Can you work these out from the model? Positions are in its coordinate system, mm. A direction names the side the tool comes from. Give positions to 0.01 mm unless a question says otherwise; leave off trailing zeros. Order: outer loops, then holes, each group sorted by start corner. A loop starts at its lowest first (then second) coordinate and runs counter-clockwise, first axis right, second up. Notation, with made-up numbers: (78.5, 6) -> (91.5, 6) arc R30 ccw to (91.5, 29) -> close; hole circle Ø4 at (-18.5, 7.5). An arc over 180 degrees is marked (long way). Answer as CSV lines item,"result".
```python
from build123d import *

# Parameters (mm, degrees)
SKETCH1_W           = 300.101088838
SKETCH1_H           = 6.35
BOSS_EXTRUDE1_DEPTH = 38.1
SKETCH2_W           = 40
SKETCH2_H           = 20
CUT_EXTRUDE1_DEPTH  = 7.35


with BuildPart() as part:
    # Sketch1 → Boss-Extrude1 (new body)
    with BuildSketch(Plane.XY.offset(-6.35)):
        with Locations((245.392650566, 49.505069687)):
            Rectangle(SKETCH1_W, SKETCH1_H)
    extrude(amount=BOSS_EXTRUDE1_DEPTH)

    # Sketch2 → Cut-Extrude1 (cut, through all)
    with BuildSketch(Plane(origin=(0, 52.680069687, 0), x_dir=(1, 0, 0), z_dir=(0, 1, 0))):
        with Locations((325.026890103, -12.7)):
            Rectangle(SKETCH2_W, SKETCH2_H)
    extrude(amount=-CUT_EXTRUDE1_DEPTH, mode=Mode.SUBTRACT)


solid = part.part
```
Item 1: Imagine slicing it at B-B, the plane x = 327. Please give me the cut outline in (y, z), then the cut area to 3 significant figures.
Numbers:
outline,"(46.33, -6.35) -> (52.68, -6.35) -> (52.68, 2.7) -> (46.33, 2.7) -> close; (46.33, 22.7) -> (52.68, 22.7) -> (52.68, 31.75) -> (46.33, 31.75) -> close"
area,"115 mm²"
Item 2: For faces 5 (the flat face through (345.027, 50, 13)), 6 (the flat face through (243, 52.68, 12)), which set-ups out of +Z, -Z, +X, -X, +Y, -Y let a thin tool reach every point of the face, with its end or its side?
Numbers:
face 5,"+Y, -Y"
face 6,"+Z, -Z, +X, -X, +Y"
Item 3: Please list where these lines run through material, in increasing order: line 1 along X through (y, z) = (51.5, 10); line 2 along Z through (x, y) = (315, 47).
Numbers:
line 1,"x = 95.34 to 305.03, 345.03 to 395.44"
line 2,"z = -6.35 to 2.7, 22.7 to 31.75"
Item 4: We'd pull the mould along Z, two halves only. Please class faces 1 (the flat face through (243, 50, 31.75)), 2 (the flat face through (243, 50, -6.35)), 3 (the flat face through (305.027, 50, 13)), 4 (the flat face through (243, 46.33, 12)): released by +Z, released by -Z, zero draft, split by the parting line, or undercut.
Numbers:
face 1,"released by +Z"
face 2,"released by -Z"
face 3,"undercut"
face 4,"zero draft"
Item 5: Imagine slicing it at A-A, the plane z = 7.5. Please give me the cut outline in (x, y), then the cut area to 3 significant figures.
Numbers:
outline,"(95.34, 46.33) -> (305.03, 46.33) -> (305.03, 52.68) -> (95.34, 52.68) -> close; (345.03, 46.33) -> (395.44, 46.33) -> (395.44, 52.68) -> (345.03, 52.68) -> close"
area,"1,650 mm²"
Item 6: Imagine slicing it at C-C, the plane y = 47.5. Please give me the cut outline in (x, z), then the cut area to 3 significant figures.
Numbers:
outline,"(95.34, -6.35) -> (395.44, -6.35) -> (395.44, 31.75) -> (95.34, 31.75) -> close; hole (305.03, 2.7) -> (345.03, 2.7) -> (345.03, 22.7) -> (305.03, 22.7) -> close"
area,"10,600 mm²"
Item 7: For pin 1 (12 mm diameter, centred on x = 324.5, z = 11, fed in from +Y), with a flat end and sliding along its axis, tell me the tip position at first contact or that it passes through.
Numbers:
pin 1,"passes through"
